Design review of the part built by this model. Coordinates are the model's own, in mm. Face numbers are marked on the shaded views. A direction names the side the tool comes from. Give positions to 0.01 mm unless a question says otherwise; leave off trailing zeros. Loops run counter-clockwise (first coordinate to the right, second up) from the corner with the lowest first, then second, coordinate; pieces in that order, holes last. Notation, with made-up numbers: (86, 70.5) -> (97, 70.5) arc R16 ccw to (97, 93.5) -> close; hole circle Ø6 at (55, 11). An arc over 180 degrees is marked (long way). Use a Markdown table: item, result. Add a question column.
1. Add section B-B (z = 12.75). State the section outline as (x, y) points.
2. Add section D-D (y = -21.5). State the section outline as (x, z) points, and give its area (3 significant figures).
3. For pin 1 Ø3 at (x, z) = (-3.5, 4.5) entering from -Y; pin 2 Ø2 at (y, z) = (-22.5, 19) entering from -X; pin 3 Ø7 at (x, y) = (-2.5, 2) entering from +Z; pin 4 Ø1.3 at (x, z) = (-18.5, 0.5) entering from -Y, all flat-tipped, find the tip position at first contact; note any pin that passes through.
4. Draft analysis for pull direction Y (two halves, no side actions). For the marked faces 1, 2 and 3, state which applies: pulls with the +Y half, pulls with the -Y half, needs draft (parallel to the pull), parting line crosses it, or undercut.
5. For the marked faces 4 and 5, list the 3-axis set-ups (+Z, -Z, +X, -X, +Y, -Y) from which the entire face can be reached by the end or side of a thin tool; tool diameter is ignored.
6. Add section C-C (x = -21). State the section outline as (y, z) points, and give its area (3 significant figures).
7. To check wall thickness, follow line 1 (X direction, y = -24.5, z = 12.5); line 2 (Z direction, x = -27, y = -6); line 3 (Z direction, x = -50, y = -16.5). State the ranges of each line that lie inside material, in increasing order.
8. Add section A-A (x = -44). State the section outline as (y, z) points, and give its area (3 significant figures).
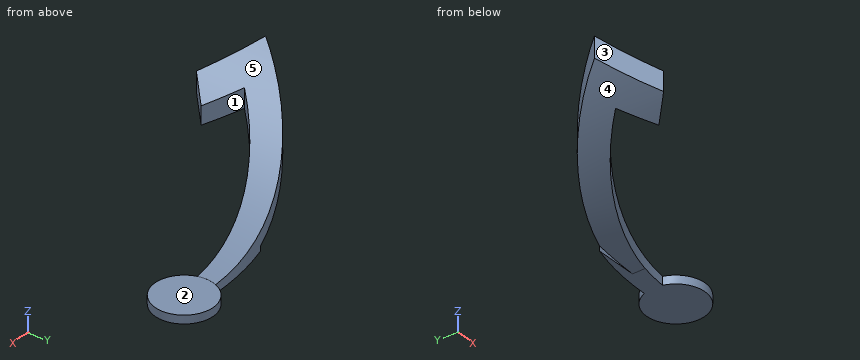
```python
from build123d import *

# Parameters (mm, degrees)
ESQUISSE3_R                  = 7
BOSS_EXTRU_2_DEPTH           = 2
BOSS_EXTRU_3_DEPTH           = 45
ENL_V_MAT_EXTRU_3_DEPTH      = 5
ENL_V_MAT_EXTRU_3_DEPTH_BACK = 81.143689392
ENL_V_MAT_EXTRU_4_DEPTH      = 70.76004634


with BuildPart() as part:
    # Esquisse3 → Boss.-Extru.2 (new body)
    with BuildSketch(Plane.XY):
        Circle(ESQUISSE3_R)
    extrude(amount=BOSS_EXTRU_2_DEPTH)

    # Esquisse3_3 → Boss.-Extru.3 (add)
    with BuildSketch(Plane.XY):
        with BuildLine():
            ThreePointArc((-6.556240583, 2.452694319), (-35.156121343, -4.82839961), (-56.806558544, -24.883974331))
            Line((-56.806558544, -24.883974331), (-47.470277823, -34.220255052))
            Line((-47.470277823, -34.220255052), (-42.209094679, -28.959071907))
            Line((-42.209094679, -28.959071907), (-48.061618993, -23.106547593))
            ThreePointArc((-48.061618993, -23.106547593), (-29.360618565, -8.682127194), (-6.699170831, -2.030051767))
            ThreePointArc((-6.699170831, -2.030051767), (-6.99644453, 0.22307834), (-6.556240583, 2.452694319))
        make_face()
    extrude(amount=BOSS_EXTRU_3_DEPTH)

    # Esquisse4 → Enl_v. mat.-Extru.3 (cut, two sides: drawn at the far end of the back side and taken through both)
    with BuildSketch(Plane(origin=(0, 0, 0), x_dir=(1, 0, 0), z_dir=(0, 1, 0)).offset(-ENL_V_MAT_EXTRU_3_DEPTH_BACK)):
        with BuildLine():
            Line((-6.556240583, -21.643777245), (-6.556240583, -2))
            ThreePointArc((-6.556240583, -2), (-33.331448935, -7.600933328), (-56.806558544, -21.643777245))
            Line((-56.806558544, -21.643777245), (-56.806558544, -45))
            Line((-56.806558544, -45), (-56.806558544, -53.527020644))
            Line((-56.806558544, -53.527020644), (-6.425184121, -53.527020644))
            Line((-6.425184121, -53.527020644), (-6.556240583, -21.643777245))
        make_face()
    extrude(amount=ENL_V_MAT_EXTRU_3_DEPTH + ENL_V_MAT_EXTRU_3_DEPTH_BACK, mode=Mode.SUBTRACT)

    # Esquisse4_4 → Enl_v. mat.-Extru.4 (cut, through all)
    with BuildSketch(Plane(origin=(0, 0, 0), x_dir=(1, 0, 0), z_dir=(0, 1, 0))):
        with BuildLine():
            ThreePointArc((-56.806558544, -16.643777245), (-36.412027531, -4.815736188), (-13.332856502, 0))
            Line((-13.332856502, 0), (-56.806558544, 0))
            Line((-56.806558544, 0), (-56.806558544, -16.643777245))
        make_face()
    extrude(amount=-ENL_V_MAT_EXTRU_4_DEPTH, mode=Mode.SUBTRACT)


solid = part.part
```
Taken from the geometry:
| question | item | result |
|---|---|---|
| 1 | outline | (-51.59, -30.1) -> (-47.47, -34.22) -> (-44.12, -30.87) -> (-44.12, -27.04) -> (-48.06, -23.11) arc R63.94 cw to (-44.12, -19.06) -> (-44.12, -10.81) arc R59.89 ccw to (-51.59, -17.98) -> close |
| 2 | outline | (-54.45, 14.79) arc R74.03 ccw to (-46.58, 9.62) -> (-46.58, 14.2) arc R82.56 cw to (-54.45, 19.71) -> close |
| 2 | area | 37.4 mm^2 |
| 3 | pin 1 | passes through |
| 3 | pin 2 | stops at x = -55.88 |
| 3 | pin 3 | stops at z = 2 |
| 3 | pin 4 | stops at y = -4.54 |
| 4 | face 1 | undercut |
| 4 | face 2 | needs draft |
| 4 | face 3 | pulls with the -Y half |
| 5 | face 4 | -Z, -X, -Y |
| 5 | face 5 | +Z, +X, +Y, -Y |
| 6 | outline | (-5.15, 0.75) -> (0, 0.75) -> (0, 0) -> (0.68, 0) -> (0.68, 3.86) -> (-5.15, 3.86) -> close |
| 6 | area | 18.6 mm^2 |
| 7 | line 1 | x = -51.22 to -46.67 |
| 7 | line 2 | z = 1.91 to 5.42 |
| 7 | line 3 | z = 11.7 to 16.43 |
| 8 | outline | (-30.75, 8.22) -> (-27.17, 8.22) -> (-27.17, 12.68) -> (-30.75, 12.68) -> close; (-18.95, 8.22) -> (-10.71, 8.22) -> (-10.71, 12.68) -> (-18.95, 12.68) -> close |
| 8 | area | 52.7 mm^2 |
